from build123d import *

# Parameters (mm, degrees)
SKETCH1_R           = 4.7625
BOSS_EXTRUDE1_DEPTH = 4.7625
SKETCH2_R           = 1.7018
CUT_EXTRUDE1_DEPTH  = 21.853960742


with BuildPart() as part:
    # Sketch1 → Boss-Extrude1 (new, symmetric)
    with BuildSketch(Plane.XY):
        with BuildLine():
            Line((6.35, 0), (-11.2141, 0))
            ThreePointArc((-11.2141, 0), (-15.210313974, 9.647713974), (-5.5626, 5.6515))
            Line((-5.5626, 5.6515), (-5.5626, 1.778))
            Line((-5.5626, 1.778), (6.35, 1.778))
            Line((6.35, 1.778), (6.35, 0))
        make_face()
        with Locations(Location((-11.2141, 5.6515, 0), (0, 0, 180))):
            Circle(SKETCH1_R, mode=Mode.SUBTRACT)
    extrude(amount=BOSS_EXTRUDE1_DEPTH, both=True)

    # Sketch2 → Cut-Extrude1 (cut, through all)
    with BuildSketch(Plane(origin=(0, 0, 0), x_dir=(1, 0, 0), z_dir=(0, 1, 0))):
        with Locations(Location((0, 0, 0), (0, 0, 90))):
            Circle(SKETCH2_R)
        with BuildLine():
            Line((0, -5.08), (0, -11.820740926))
            Line((0, -11.820740926), (11.381105031, -11.820740926))
            Line((11.381105031, -11.820740926), (11.381105031, 11.820740926))
            Line((11.381105031, 11.820740926), (0, 11.820740926))
            Line((0, 11.820740926), (0, 5.08))
            ThreePointArc((0, 5.08), (5.08, 0), (0, -5.08))
        make_face()
    extrude(amount=CUT_EXTRUDE1_DEPTH, mode=Mode.SUBTRACT)


solid = part.part
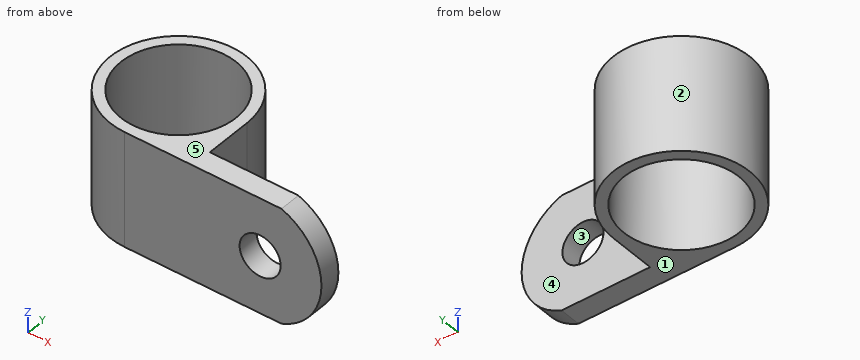
For this review, take the finished solid that the model builds, in its own axes (mm). Face numbers are marked on the shaded views. A direction names the side the tool comes from. Give positions to 0.01 mm unless a question says otherwise; leave off trailing zeros. Loops run counter-clockwise (first coordinate to the right, second up) from the corner with the lowest first, then second, coordinate; pieces in that order, holes last.
Item 1: Take a section at A-A, the plane z = 0. State the section outline as (x, y) points (1 decimal), and give its area (3 significant figures).
Item 2: Take a section at B-B, the plane x = 0. State the section outline as (y, z) points, and give its area (3 significant figures).
Item 3: Take a section at C-C, the plane y = 7.25. State the section outline as (x, z) points.
Item 4: Tool access review of the marked faces 4 and 5: name each direction out of +Z, -Z, +X, -X, +Y, -Y from which nothing blocks a thin tool from reaching the whole face with its end or side.
Item 5: Insertion check: pin 1 (5 mm diameter, centred on y = 5, z = 1, fed in from +X); pin 2 (3 mm diameter, centred on x = -1, z = -2, fed in from +Y); pin 3 (1.5 mm diameter, centred on y = 1.5, z = -1, fed in from +X). Each pin has a flat end and moves straight along its axis. Give the tip position at first contact, or say it passes through.
Item 6: Take a section at D-D, the plane z = 2.25. State the section outline as (x, y) points (1 decimal).
Item 7: Draft analysis for pull direction Z (two halves, no side actions). For the marked faces 1, 2 and 3, state which applies: +Z half, -Z half, draft (parallel to the pull), parting line (faces both ways), or undercut.
Item 8: For line 1 along X through (y, z) = (1.5, 0.75); line 2 along X through (y, z) = (1.45, 0); line 3 along Y through (x, z) = (0.5, 3.75), list the stretches that pass through material, from the lowest coordinate up.
Calculated:
1. outline: (-11.2, 0) - (-1.7, 0) - (-1.7, 1.8) - (-5.6, 1.8) - (-5.6, 5.7) arc R5.7 ccw (long way) to start; (1.7, 0) - (5.1, 0) - (5.1, 1.8) - (1.7, 1.8) - close; hole circle Ø9.5 at (-11.2, 5.7)
1. area: 48.8 mm2
2. outline: (0, -4.76) - (1.78, -4.76) - (1.78, -1.7) - (0, -1.7) - close; (0, 1.7) - (1.78, 1.7) - (1.78, 4.76) - (0, 4.76) - close
2. area: 10.9 mm2
3. outline: (-16.63, -4.76) - (-15.7, -4.76) - (-15.7, 4.76) - (-16.63, 4.76) - close; (-6.73, -4.76) - (-5.79, -4.76) - (-5.79, 4.76) - (-6.73, 4.76) - close
4. face 4: +Z, -Z, +X, +Y
4. face 5: +Z, +X, -X, +Y, -Y
5. pin 1: stops at x = -5.56
5. pin 2: stops at y = 1.78
5. pin 3: stops at x = 5.07
6. outline: (-11.2, 0) - (4.6, 0) - (4.6, 1.8) - (-5.6, 1.8) - (-5.6, 5.7) arc R5.7 ccw (long way) to start; hole circle Ø9.5 at (-11.2, 5.7)
7. face 1: -Z half
7. face 2: draft
7. face 3: undercut
8. line 1: x = -15.05 to -13.55, -8.88 to -1.53, 1.53 to 5.02
8. line 2: x = -14.99 to -13.46, -8.97 to -1.7, 1.7 to 5.08
8. line 3: y = 0 to 1.78
